Part model, mm, in its own coordinate system. A direction names the side the tool comes from. Round coordinates to 2 decimals unless told otherwise and drop trailing zeros. Loops run counter-clockwise (first coordinate to the right, second up) from the corner with the lowest first, then second, coordinate; pieces in that order, holes last.
1) Drop flat-ended pins along their axis: P1, Ø12, axis at x = -25, z = 24, coming from the -Y side; P2, Ø3, axis at x = -13.5, y = 65, coming from the -Z side; P3, Ø17, axis at x = -15, y = 41, coming from the +Z side; P4, Ø15.5, axis at x = -20, z = 34, coming from the +Y side. Give the stop position or say it passes through.
2) 3-axis set-ups, long thin cutter, end or side, ignore diameter. For faces 5 (the flat face through (-20, 58, 7)), 6 (the flat face through (-20, 10, 10)), 7 (the flat face through (-20, 40, 10)): which of +Z, -Z, +X, -X, +Y, -Y reach the whole face in a straight line?
3) Probe line 1 (X direction, y = 63.25, z = 34); line 2 (Z direction, x = -20, y = 54); line 3 (Y direction, x = -37, z = 20.5). List the from-to ranges inside material, lowest first.
4) Band-saw the part on A-A, the plane z = 34. Write the cut outline in (x, y), then the cut area to 3 significant figures.
5) Mould opens along Z. For faces 1 (the flat face through (-20, 59, 54)), 2 (the flat face through (-6, 68, 34)), 3 (the cylindrical face through (-19.428, 58.874, 46.987)), 4 (the flat face through (-20, 63, 14)) say: +Z half, -Z half, draft (parallel to the pull), parting line (faces both ways), or undercut.
6) Band-saw the part on C-C, the plane x = -20. Write the cut outline in (y, z), then the cut area to 3 significant figures.
7) Band-saw the part on B-B, the plane y = 52.5. Write the cut outline in (x, z), then the cut area to 3 significant figures.
8) Band-saw the part on D-D, the plane x = -36.5. Write the cut outline in (y, z), then the cut area to 3 significant figures.
Solid Edge part; units mm, degrees
sketch "Sketch1" plane through (0, 0, 0) normal (1, 0, 0) x (0, 1, 0)
  line L0 (19, 22) -> (19, 10)
  line L1 (19, 10) -> (0, 10)
  line L2 (0, 10) -> (0, 0)
  line L3 (0, 0) -> (58, 0)
  line L4 (58, 0) -> (58, 14)
  line L5 (58, 14) -> (68, 14)
  line L6 (68, 14) -> (68, 54)
  line L7 (68, 54) -> (50, 54)
  line L8 (50, 54) -> (50, 10)
  line L9 (50, 10) -> (29, 10)
  line L10 (29, 10) -> (29, 22)
  line L11 (29, 22) -> (19, 22)
extrude "ProtrusiónExtruida_1" add sketch "Sketch1" against normal blind 40
hole "Agujero_1" at (-20, 50, 34) direction (0, 1, 0) diameter 26 end up to next
Reported:
1. P1: stops at y = 19
1. P2: stops at z = 14
1. P3: stops at z = 10
1. P4: passes through
2. face 5: -Z, +X, -X, +Y
2. face 6: +Z, +X, -X, -Y
2. face 7: +Z, +X, -X
3. line 1: x = -40 to -33, -7 to 0
3. line 2: z = 0 to 21, 47 to 54
3. line 3: y = 19 to 29, 50 to 68
4. outline: (-40, 50) - (-33, 50) - (-33, 68) - (-40, 68) - close; (-7, 50) - (0, 50) - (0, 68) - (-7, 68) - close
4. area: 252 mm2
5. face 1: +Z half
5. face 2: draft
5. face 3: undercut
5. face 4: -Z half
6. outline: (0, 0) - (58, 0) - (58, 14) - (68, 14) - (68, 21) - (50, 21) - (50, 10) - (29, 10) - (29, 22) - (19, 22) - (19, 10) - (0, 10) - close; (50, 47) - (68, 47) - (68, 54) - (50, 54) - close
6. area: 984 mm2
7. outline: (-40, 0) - (0, 0) - (0, 54) - (-40, 54) - close; hole circle Ø26 at (-20, 34)
7. area: 1,630 mm2
8. outline: (0, 0) - (58, 0) - (58, 14) - (68, 14) - (68, 54) - (50, 54) - (50, 10) - (29, 10) - (29, 22) - (19, 22) - (19, 10) - (0, 10) - close
8. area: 1,450 mm2
